The listing builds one solid part. Answer for the finished solid, in the listing's coordinates (mm). A direction names the side the tool comes from. Coordinates: 2 decimals unless noted, no trailing zeros. Write each loop counter-clockwise with the first axis right and the second up, starting at its lowest first coordinate (ties: lowest second). Pieces come first, ordered by that corner, then holes.
(1) Which of the six approach directions +Z, -Z, +X, -X, +Y, -Y give full straight-line access (tool end or side, diameter ignored) to faces 1 (the cylindrical face through (-7.32, 99.11, 1.52)), 2 (the cylindrical face through (25.03, 99.28, 1.48)), 3 (the flat face through (49, 154, 0))?
(2) The part is cut by section B-B on z = 0.5. Give the number of separate pieces and of enclosed holes in the cut face, plus the area to 3 significant figures.
(3) Straight lines are drawn through the part: line 1 (Y direction, x = 12.5, z = 1.25); line 2 (Y direction, x = 24.5, z = 2.65); line 3 (Y direction, x = 16.5, z = 1.6). For each, find the intervals that lie inside material, in ascending order.
(4) For a pull along X with two mould halves and no side action, classify faces 4 (the cylindrical face through (-7.15, -7.99, 1.52)), 5 (the cylindrical face through (-0.59, 4.46, 1.48)), 6 (the flat face through (30.2, 10.2, 1.5)) as +X half, -X half, draft (parallel to the pull), parting line (faces both ways), or undercut.
(5) Given P1, Ø2.5, axis at x = 75.7, y = 195.11, coming from the -Z side, flat-ended and moving along its own axis, determine where the tip first touches the part or whether it passes through.
(6) The part is cut by section A-A on y = 311. Determine the outline of the cut face in (x, z).
from build123d import *

# Parameters (mm, degrees)
SKETCH_1_W          = 20
SKETCH_1_H          = 60
SKETCH_1_R          = 4.5
EXTRUDE_1_DEPTH     = 3
EXTRUDE_START       = -3
EXTRUDE_2_DEPTH     = 3
FILLET_2_R          = 20
FILLET_3_R          = 10
FILLET_4_R          = 3
FILLET_5_R          = 10
CUT_EXTRUDE_1_DEPTH = 384.952760264
CUT_EXTRUDE_2_DEPTH = 384.952760264
SKETCH_5_R          = 1.5
CUT_EXTRUDE_3_DEPTH = 384.952760264
CUT_EXTRUDE_4_DEPTH = 384.952760264
EXTRUDE_3_DEPTH     = 3
FILLET_6_R          = 10
FILLET_7_R          = 5
SKETCH_8_R          = 1.5
CUT_EXTRUDE_5_DEPTH = 384.952760264


with BuildPart() as part:
    # 草图1 → 凸台-拉伸1 (new body)
    # profile 1 of 4: a face of its own
    with BuildSketch(Plane.XY):
        with BuildLine():
            ThreePointArc((88, 226.5), (59.064327086, 318.272229816), (-17.276777068, 376.850819326))
            Line((-17.276777068, 376.850819326), (-24.117179934, 358.05696691))
            ThreePointArc((-24.117179934, 358.05696691), (42.6812862, 306.800701089), (68, 226.5))
            ThreePointArc((68, 226.5), (52.659536338, 162.781870712), (10, 113.02753638))
            Line((10, 113.02753638), (10, 89.110044035))
            ThreePointArc((10, 89.110044035), (67.140217047, 147.506329367), (88, 226.5))
        make_face()
    # profile 2 of 4: a face of its own
    with BuildSketch(Plane.XY):
        with BuildLine():
            Line((-10, 100.977093724), (-10, 79.00084746))
            ThreePointArc((-10, 79.00084746), (0.177205293, 83.704863402), (10, 89.110044035))
            Line((10, 89.110044035), (10, 113.02753638))
            ThreePointArc((10, 113.02753638), (0.251666362, 106.584626891), (-10, 100.977093724))
        make_face()
    # profile 3 of 4: a face of its own
    with BuildSketch(Plane.XY):
        with BuildLine():
            Line((-10, 79.00084746), (-10, 49))
            Line((-10, 49), (10, 49))
            Line((10, 49), (10, 89.110044035))
            ThreePointArc((10, 89.110044035), (0.177205293, 83.704863402), (-10, 79.00084746))
        make_face()
    # profile 4 of 4: a face of its own
    with BuildSketch(Plane.XY):
        with Locations((0, 19)):
            Rectangle(SKETCH_1_W, SKETCH_1_H)
        with Locations((0, 38)):
            Circle(SKETCH_1_R, mode=Mode.SUBTRACT)
        Circle(SKETCH_1_R, mode=Mode.SUBTRACT)
    extrude(amount=EXTRUDE_1_DEPTH)

    # 草图2 → 凸台-拉伸2 (add)
    with BuildSketch(Plane.XY.offset(3).offset(EXTRUDE_START)):
        with BuildLine():
            Line((10, -1), (10, -11))
            Line((10, -11), (40, -11))
            Line((40, -11), (84.331190721, 192.433024677))
            ThreePointArc((84.331190721, 192.433024677), (74.827433124, 162.925595698), (59.811855282, 135.804714527))
            Line((59.811855282, 135.804714527), (30, -1))
            Line((30, -1), (10, -1))
        make_face()
    extrude(amount=EXTRUDE_2_DEPTH)

    # 圆角2
    fillet_2_edges = [part.edges().sort_by_distance(p)[0] for p in [
        (-10, 100.977093724, 1.5),
    ]]
    fillet(fillet_2_edges, radius=FILLET_2_R)

    # 圆角3
    fillet_3_edges = [part.edges().sort_by_distance(p)[0] for p in [
        (-10, -11, 1.5),
        (40, -11, 1.5),
    ]]
    fillet(fillet_3_edges, radius=FILLET_3_R)

    # 圆角4
    fillet_4_edges = [part.edges().sort_by_distance(p)[0] for p in [
        (-24.117179934, 358.05696691, 1.5),
    ]]
    fillet(fillet_4_edges, radius=FILLET_4_R)

    # 圆角5
    fillet_5_edges = [part.edges().sort_by_distance(p)[0] for p in [
        (-17.276777068, 376.850819326, 1.5),
    ]]
    fillet(fillet_5_edges, radius=FILLET_5_R)

    # 草图3 → 切除-拉伸1 (cut, through all)
    with BuildSketch(Plane(origin=(0, 0, 0), x_dir=(-1, 0, 0), z_dir=(0, 0, -1))):
        Polygon((-46.77842194, 43.588901874), (-43.847212114, 44.227657662), (-42.143863348, 36.411098126), (-45.075073174, 35.772342338), align=None)
        Polygon((-70.199467474, 151.066595495), (-68.496118708, 143.250035959), (-65.564908882, 143.888791747), (-67.268257648, 151.705351283), align=None)
    extrude(amount=-CUT_EXTRUDE_1_DEPTH, mode=Mode.SUBTRACT)

    # 草图4 → 切除-拉伸2 (cut, through all)
    with BuildSketch(Plane(origin=(0, 0, 0), x_dir=(-1, 0, 0), z_dir=(0, 0, -1))):
        Polygon((-28.272186631, 109.750418514), (-28.533653859, 112.739002608), (-20.564096275, 113.43624855), (-20.302629046, 110.447664456), align=None)
        Polygon((-81.889087297, 228.267766953), (-76.232233047, 222.610912703), (-74.110912703, 224.732233047), (-79.767766953, 230.389087297), align=None)
        Polygon((-25.563810529, 345.522178874), (-26.261056471, 337.55262129), (-23.272472377, 337.291154061), (-22.575226435, 345.260711646), align=None)
        Polygon((100.463470173, 377.744196764), (93.910253818, 373.155585273), (95.630983127, 370.69812914), (102.184199482, 375.286740631), align=None)
    extrude(amount=-CUT_EXTRUDE_2_DEPTH, mode=Mode.SUBTRACT)

    # 草图5 → 切除-拉伸3 (cut, through all)
    with BuildSketch(Plane.XY.offset(3)):
        with Locations((72.125207072, 166.801384551)):
            Circle(SKETCH_5_R)
        with Locations((75.700287711, 195.105334687)):
            Circle(SKETCH_5_R)
        with Locations(Location((54.63925576, 144.259505713, 0), (0, 0, 180))):
            Circle(SKETCH_5_R)
        with Locations(Location((34.773123959, 333.273123959, 0), (0, 0, 180))):
            Circle(SKETCH_5_R)
        with Locations((16.35937296, 355.063685425)):
            Circle(SKETCH_5_R)
        with Locations((-10.582766896, 364.445364104)):
            Circle(SKETCH_5_R)
    extrude(amount=-CUT_EXTRUDE_3_DEPTH, mode=Mode.SUBTRACT)

    # 草图6 → 切除-拉伸4 (cut, through all)
    with BuildSketch(Plane(origin=(0, 0, 0), x_dir=(-1, 0, 0), z_dir=(0, 0, -1))):
        Polygon((-48.895829905, 29.822399649), (-37.268809589, 32.356106534), (-10, -1), (-10, -25.455905849), (-44.544329985, -23.840605691), align=None)
    extrude(amount=-CUT_EXTRUDE_4_DEPTH, mode=Mode.SUBTRACT)

    # 草图7 → 凸台-拉伸3 (add)
    with BuildSketch(Plane(origin=(0, 0, 0), x_dir=(-1, 0, 0), z_dir=(0, 0, -1))):
        Polygon((-48.895829905, 29.822399649), (-10, -11), (-10, 6.39592954), (-38.020150061, 35.803960345), (-37.268809589, 32.356106534), align=None)
    extrude(amount=-EXTRUDE_3_DEPTH)

    # 圆角6
    fillet_6_edges = [part.edges().sort_by_distance(p)[0] for p in [
        (10, 89.110044035, 1.5),
        (10, -11, 1.5),
        (48.895829905, 29.822399649, 1.5),
        (59.811855282, 135.804714527, 1.5),
    ]]
    fillet(fillet_6_edges, radius=FILLET_6_R)

    # 圆角7
    fillet_7_edges = [part.edges().sort_by_distance(p)[0] for p in [
        (38.020150061, 35.803960345, 1.5),
        (10, 6.39592954, 1.5),
    ]]
    fillet(fillet_7_edges, radius=FILLET_7_R)

    # 草图8 → 切除-拉伸5 (cut, through all)
    with BuildSketch(Plane(origin=(0, 0, 0), x_dir=(-1, 0, 0), z_dir=(0, 0, -1))):
        with Locations((-43.609468261, 36.091720232)):
            Circle(SKETCH_8_R)
        with Locations((-45.312817027, 43.908279768)):
            Circle(SKETCH_8_R)
        with Locations((-67.030513795, 143.569413853)):
            Circle(SKETCH_8_R)
        with Locations((-68.733862561, 151.385973389)):
            Circle(SKETCH_8_R)
        with Locations((-28.402920245, 111.244710561)):
            Circle(SKETCH_8_R)
        with Locations((-20.433362661, 111.941956503)):
            Circle(SKETCH_8_R)
        with Locations((-75.171572875, 223.671572875)):
            Circle(SKETCH_8_R)
        with Locations((-80.828427125, 229.328427125)):
            Circle(SKETCH_8_R)
        with Locations((-24.766764424, 337.421887675)):
            Circle(SKETCH_8_R)
        with Locations((-24.069518482, 345.39144526)):
            Circle(SKETCH_8_R)
    extrude(amount=-CUT_EXTRUDE_5_DEPTH, mode=Mode.SUBTRACT)


solid = part.part
Model answer:
1. face 1: +Z, -Z, -X
1. face 2: +Z, -Z
1. face 3: -Z, +X, -X, +Y, -Y
2. separate pieces: 1
2. enclosed holes: 14
2. area: 10,900 mm2
3. line 1: y = -8.35 to 14.56, 90.16 to 114.88, 338.12 to 362.37
3. line 2: y = 4.22 to 21.61, 98.88 to 110.08, 113.09 to 125.07, 327.93 to 335.95, 346.83 to 354.12
3. line 3: y = -4.18 to 14.12, 93.2 to 118.02, 334.98 to 353.57, 356.56 to 359.8
4. face 4: -X half
4. face 5: undercut
4. face 6: +X half
5. P1: passes through
6. outline: (39.62, 0) - (63.87, 0) - (63.87, 3) - (39.62, 3) - close
